from build123d import *

# Parameters (mm, degrees)
SKETCH1_W                    = 84.8
SKETCH1_H                    = 93
SKETCH1_R                    = 2
BOSS_EXTRUDE1_DEPTH          = 4.7625
FILLET1_R                    = 3.18
F_6_0_6_DIAMETER_HOLE1_D     = 6
F_6_0_6_DIAMETER_HOLE1_DEPTH = 24
F_6_0_6_DIAMETER_HOLE1_TIP   = 1.802581857
CHAMFER1_SIZE                = 2
M5X0_8_TAPPED_HOLE1_D        = 4.2
M5X0_8_TAPPED_HOLE1_DEPTH    = 14
M5X0_8_TAPPED_HOLE1_TIP      = 1.2618073


with BuildPart() as part:
    # Sketch1 → Boss-Extrude1 (new body)
    with BuildSketch(Plane.XY):
        with Locations((0, 13)):
            Rectangle(SKETCH1_W, SKETCH1_H)
        with Locations(Location((15, -19, 0), (0, 0, 180))):
            Circle(SKETCH1_R, mode=Mode.SUBTRACT)
        with Locations(Location((-15, -19, 0), (0, 0, 180))):
            Circle(SKETCH1_R, mode=Mode.SUBTRACT)
        with Locations(Location((15, 19, 0), (0, 0, 180))):
            Circle(SKETCH1_R, mode=Mode.SUBTRACT)
        with Locations(Location((-15, 19, 0), (0, 0, 180))):
            Circle(SKETCH1_R, mode=Mode.SUBTRACT)
    extrude(amount=BOSS_EXTRUDE1_DEPTH)

    # Fillet1
    fillet1_edges = [part.edges().sort_by_distance(p)[0] for p in [
        (-42.4, -33.5, 2.38125),
        (-42.4, 59.5, 2.38125),
        (42.4, 59.5, 2.38125),
        (42.4, -33.5, 2.38125),
    ]]
    fillet(fillet1_edges, radius=FILLET1_R)

    # Ø6.0 (6) Diameter Hole1
    with Locations(Plane(origin=(0, 0, 0), x_dir=(-1, 0, 0), z_dir=(0, 0, -1))):
        with Locations((0, 51.5), (0.336501066, 35.75)):
            Hole(F_6_0_6_DIAMETER_HOLE1_D / 2, depth=F_6_0_6_DIAMETER_HOLE1_DEPTH)
            with Locations((0, 0, -(F_6_0_6_DIAMETER_HOLE1_DEPTH + F_6_0_6_DIAMETER_HOLE1_TIP / 2))):  # 118° drill point
                Cone(0, F_6_0_6_DIAMETER_HOLE1_D / 2, F_6_0_6_DIAMETER_HOLE1_TIP, mode=Mode.SUBTRACT)

    # Chamfer1
    chamfer1_edges = [part.edges().sort_by_distance(p)[0] for p in [
        (-13, -19, 4.7625),
        (17, 19, 4.7625),
        (-13, 19, 4.7625),
        (17, -19, 4.7625),
    ]]
    chamfer(chamfer1_edges, length=CHAMFER1_SIZE)

    # M5x0.8 Tapped Hole1
    with Locations(Plane.XY.offset(4.7625)):
        with Locations((-70.208358725, 8.341624021), (-69.847000611, 8.341624021), (-25, 5.982129573), (-5, 5.982129573)):
            Hole(M5X0_8_TAPPED_HOLE1_D / 2, depth=M5X0_8_TAPPED_HOLE1_DEPTH)
            with Locations((0, 0, -(M5X0_8_TAPPED_HOLE1_DEPTH + M5X0_8_TAPPED_HOLE1_TIP / 2))):  # 118° drill point
                Cone(0, M5X0_8_TAPPED_HOLE1_D / 2, M5X0_8_TAPPED_HOLE1_TIP, mode=Mode.SUBTRACT)


solid = part.part
The model under review builds one solid part; all positions refer to its coordinate system, in mm. Give positions to 0.01 mm unless a question says otherwise; leave off trailing zeros. Write each loop counter-clockwise with the first axis right and the second up, starting at its lowest first coordinate (ties: lowest second). Pieces come first, ordered by that corner, then holes.
1. For P1, Ø3.5, axis at x = 15, y = 19, coming from the -Z side; P2, Ø8, axis at x = 0, y = 51.5, coming from the -Z side; P3, Ø5, axis at x = -15, y = 19, coming from the +Z side, all flat-tipped, find the tip position at first contact; note any pin that passes through.
2. Add section C-C, the plane y = -19. Write out the cut boundary in (x, z), plus the area to 3 significant figures.
3. Draft analysis for pull direction Y (two halves, no side actions). For faces 1 (the cylindrical face through (-41.493, -32.544, 2.415)), 2 (the cylindrical face through (-15, 17, 1)), 3 (the flat face through (42.4, 12, 2)), state which applies: +Y half, -Y half, draft (parallel to the pull), parting line (faces both ways), or undercut.
4. Add section D-D, the plane x = -15. Write out the cut boundary in (y, z).
5. Wall thickness on L1, parallel to Y at x = 0, z = 2.5; L2, parallel to Y at x = 15, z = 0.65; L3, parallel to X at y = -19, z = 2.15: over which ranges is each line inside the solid? List them lowest first.
6. Add section B-B, the plane x = -5. Write out the cut boundary in (y, z).
7. Add section A-A, the plane y = 35.75. Write out the cut boundary in (x, z), plus the area to 3 significant figures.
Worked answers:
1. P1: passes through
1. P2: stops at z = 0
1. P3: stops at z = 3.26
2. outline: (-42.4, 0) - (-17, 0) - (-17, 2.76) - (-19, 4.76) - (-42.4, 4.76) - close; (-13, 0) - (13, 0) - (13, 2.76) - (11, 4.76) - (-11, 4.76) - (-13, 2.76) - close; (17, 0) - (42.4, 0) - (42.4, 4.76) - (19, 4.76) - (17, 2.76) - close
2. area: 358 mm2
3. face 1: -Y half
3. face 2: undercut
3. face 3: draft
4. outline: (-33.5, 0) - (-21, 0) - (-21, 2.76) - (-23, 4.76) - (-33.5, 4.76) - close; (-17, 0) - (17, 0) - (17, 2.76) - (15, 4.76) - (-15, 4.76) - (-17, 2.76) - close; (21, 0) - (59.5, 0) - (59.5, 4.76) - (23, 4.76) - (21, 2.76) - close
5. L1: y = -33.5 to 32.77, 38.73 to 48.5, 54.5 to 59.5
5. L2: y = -33.5 to -21, -17 to 17, 21 to 59.5
5. L3: x = -42.4 to -17, -13 to 13, 17 to 42.4
6. outline: (-33.5, 0) - (3.88, 0) - (3.88, 4.76) - (-33.5, 4.76) - close; (8.08, 0) - (59.5, 0) - (59.5, 4.76) - (8.08, 4.76) - close
7. outline: (-42.4, 0) - (-3.34, 0) - (-3.34, 4.76) - (-42.4, 4.76) - close; (2.66, 0) - (42.4, 0) - (42.4, 4.76) - (2.66, 4.76) - close
7. area: 375 mm2
